Build history of the part. All positions in model axes, mm. A direction names the side the tool comes from. Give positions to 0.01 mm unless a question says otherwise; leave off trailing zeros. Order: outer loops, then holes, each group sorted by start corner. A loop starts at its lowest first (then second) coordinate and runs counter-clockwise, first axis right, second up. Notation, with made-up numbers: (-15, 14) - (37, 14) arc R34 cw to (37, 46) - close; hole circle Ø5 at (38, 50). An arc over 180 degrees is marked (long way). Use a Markdown table: item, result.
from build123d import *

# Parameters (mm, degrees)
F0_W          = 10
F0_H          = 15
F1_DEPTH      = 8
F2_W          = 8
F2_H          = 14
F3_DEPTH      = 14
F5_DEPTH      = 25
F7_DEPTH      = 1
F8_R          = 2
F9_DEPTH      = 1
F10_T1_DEPTH  = 4
F10_S5_W      = 2.04
F10_S5_H      = 2.04
F10_T6_DEPTH  = 2.04
F10_S11_W     = 2.04
F10_S11_H     = 2.04
F10_T12_DEPTH = 2.04
F10_T18_DEPTH = 10
F10_T23_DEPTH = 10
F10_T28_DEPTH = 17
F10_T33_DEPTH = 17
F10_T35_DEPTH = 6
F10_T37_DEPTH = 18
F10_T39_DEPTH = 11
F10_S43_W     = 2.04
F10_S43_H     = 2.04
F10_T44_DEPTH = 2.04
F10_S49_W     = 2.04
F10_S49_H     = 2.04
F10_T50_DEPTH = 2.04


# Not quite as in the source:
# - a fillet or chamfer that OpenCascade refuses, or shapes differently, is made with other operations: its cross-section is extruded or revolved along the edge and cut away or added


with BuildPart() as f1:
    # F0 (on Front) → F1 (new body)
    with BuildSketch(Plane.XZ):
        with Locations((0, 7.5)):
            Rectangle(F0_W, F0_H)
    extrude(amount=F1_DEPTH)

    # F2 (on face) → F3 (cut)
    with BuildSketch(Plane.XZ.offset(8)):
        with Locations((0, 8)):
            Rectangle(F2_W, F2_H)
    extrude(amount=-F3_DEPTH, mode=Mode.SUBTRACT)

    # F4 (on face) → F5 (cut)
    with BuildSketch(Plane(origin=(-5, 0, 0), x_dir=(0, -1, 0), z_dir=(-1, 0, 0))):
        Polygon((8, 15), (1, 15), (8, 1), align=None)
    extrude(amount=-F5_DEPTH, mode=Mode.SUBTRACT)

    # F6 (on face) → F7 (join)
    with BuildSketch(Plane(origin=(0, 0, 0), x_dir=(-1, 0, 0), z_dir=(0, 1, 0))):
        Polygon((4, 15), (5, 15), (2.1132486541, 20), (-2.1132486541, 20), (-5, 15), (-4, 15), (-4, 1), (4, 1), align=None)
    extrude(amount=-F7_DEPTH)

    # F8 (on face) → F9 (join)
    with BuildSketch(Plane.XZ.offset(1)):
        with Locations((0, 17)):
            Circle(F8_R)
    extrude(amount=F9_DEPTH)

    # F10: fillet of radius 2 on 12 edges, made by hand

    # F10_s2 → F10_t1 (join)
    with BuildSketch(Plane.YZ.offset(-2)):
        with BuildLine():
            ThreePointArc((-3, 1), (-1.5857864376, 1.5857864376), (-1, 3))
            Line((-1, 3), (-1, 1))
            Line((-1, 1), (-3, 1))
        make_face()
    extrude(amount=F10_T1_DEPTH)


with BuildPart() as f10_tool4:
    # F10_s5 → F10_t6 (new body)
    with BuildSketch(Plane.XY.offset(3)):
        with Locations((-3.02, -1.98)):
            Rectangle(F10_S5_W, F10_S5_H)
    extrude(amount=-F10_T6_DEPTH)

    # F10_s7 → F10_t8 (revolve, cut)
    with BuildSketch(Plane(origin=(-2, -3, 3), x_dir=(0.7071067812, -0.7071067812, 0), z_dir=(0.7071067812, 0.7071067812, 0))):
        with BuildLine():
            ThreePointArc((0, -2), (2, 0), (0, 2))
            Line((0, 2), (0, -2))
        make_face()
    revolve(axis=Axis((-2, -3, 3), (0, 0, -1)), mode=Mode.SUBTRACT)


with BuildPart() as f1_1:
    add(f1.part)

    # F10_t3: union F10_tool4
    add(f10_tool4.part)


with BuildPart() as f10_tool10:
    # F10_s11 → F10_t12 (new body)
    with BuildSketch(Plane.XY.offset(3)):
        with Locations((3.02, -1.98)):
            Rectangle(F10_S11_W, F10_S11_H)
    extrude(amount=-F10_T12_DEPTH)

    # F10_s13 → F10_t14 (revolve, cut)
    with BuildSketch(Plane(origin=(2, -3, 3), x_dir=(-0.7071067812, -0.7071067812, 0), z_dir=(0.7071067812, -0.7071067812, 0))):
        with BuildLine():
            ThreePointArc((0, -2), (2, 0), (0, 2))
            Line((0, 2), (0, -2))
        make_face()
    revolve(axis=Axis((2, -3, 3), (0, 0, -1)), mode=Mode.SUBTRACT)


with BuildPart() as f1_2:
    add(f1_1.part)

    # F10_t9: union F10_tool10
    add(f10_tool10.part)


with BuildPart() as f10_tool16:
    # F10_s17 → F10_t18 (new body)
    with BuildSketch(Plane.XZ.offset(13)):
        with BuildLine():
            ThreePointArc((-2, 1), (-3.4142135624, 1.5857864376), (-4, 3))
            Line((-4, 3), (-4, 1))
            Line((-4, 1), (-2, 1))
        make_face()
    extrude(amount=-F10_T18_DEPTH)

    split(bisect_by=Plane(origin=(0, -6.8, 3.4), x_dir=(1, 0, 0), z_dir=(0, 0.894427191, -0.4472135955)), keep=Keep.TOP)


with BuildPart() as f1_3:
    add(f1_2.part)

    # F10_t15: union F10_tool16
    add(f10_tool16.part)


with BuildPart() as f10_tool21:
    # F10_s22 → F10_t23 (new body)
    with BuildSketch(Plane.XZ.offset(13)):
        with BuildLine():
            ThreePointArc((2, 1), (3.4142135624, 1.5857864376), (4, 3))
            Line((4, 3), (4, 1))
            Line((4, 1), (2, 1))
        make_face()
    extrude(amount=-F10_T23_DEPTH)

    split(bisect_by=Plane(origin=(0, -6.8, 3.4), x_dir=(1, 0, 0), z_dir=(0, 0.894427191, -0.4472135955)), keep=Keep.TOP)


with BuildPart() as f1_4:
    add(f1_3.part)

    # F10_t20: union F10_tool21
    add(f10_tool21.part)


with BuildPart() as f10_tool26:
    # F10_s27 → F10_t28 (new body)
    with BuildSketch(Plane.XY.offset(20)):
        with BuildLine():
            ThreePointArc((2, -1), (3.4142135624, -1.5857864376), (4, -3))
            Line((4, -3), (4, -1))
            Line((4, -1), (2, -1))
        make_face()
    extrude(amount=-F10_T28_DEPTH)

    split(bisect_by=Plane(origin=(0, -6.8, 3.4), x_dir=(1, 0, 0), z_dir=(0, 0.894427191, -0.4472135955)), keep=Keep.TOP)


with BuildPart() as f1_5:
    add(f1_4.part)

    # F10_t25: union F10_tool26
    add(f10_tool26.part)


with BuildPart() as f10_tool31:
    # F10_s32 → F10_t33 (new body)
    with BuildSketch(Plane.XY.offset(3)):
        with BuildLine():
            ThreePointArc((-4, -3), (-3.4142135624, -1.5857864376), (-2, -1))
            Line((-2, -1), (-4, -1))
            Line((-4, -1), (-4, -3))
        make_face()
    extrude(amount=F10_T33_DEPTH)

    split(bisect_by=Plane(origin=(0, -6.8, 3.4), x_dir=(1, 0, 0), z_dir=(0, 0.894427191, -0.4472135955)), keep=Keep.TOP)


with BuildPart() as f1_6:
    add(f1_5.part)

    # F10_t30: union F10_tool31
    add(f10_tool31.part)

    # F10_s36 → F10_t35 (cut)
    with BuildSketch(Plane.YZ.offset(-3)):
        with BuildLine():
            ThreePointArc((-2, 0), (-0.5857864376, 0.5857864376), (0, 2))
            Line((0, 2), (0, 0))
            Line((0, 0), (-2, 0))
        make_face()
    extrude(amount=F10_T35_DEPTH, mode=Mode.SUBTRACT)

    # F10_s38 → F10_t37 (cut)
    with BuildSketch(Plane.XY.offset(2)):
        with BuildLine():
            ThreePointArc((-5, -2), (-4.4142135624, -0.5857864376), (-3, 0))
            Line((-3, 0), (-5, 0))
            Line((-5, 0), (-5, -2))
        make_face()
        with BuildLine():
            ThreePointArc((5, -2), (4.4142135624, -0.5857864376), (3, 0))
            Line((3, 0), (5, 0))
            Line((5, 0), (5, -2))
        make_face()
    extrude(amount=F10_T37_DEPTH, mode=Mode.SUBTRACT)

    # F10_s40 → F10_t39 (cut)
    with BuildSketch(Plane.XZ.offset(2)):
        with BuildLine():
            ThreePointArc((-5, 2), (-4.4142135624, 0.5857864376), (-3, 0))
            Line((-3, 0), (-5, 0))
            Line((-5, 0), (-5, 2))
        make_face()
        with BuildLine():
            ThreePointArc((5, 2), (4.4142135624, 0.5857864376), (3, 0))
            Line((3, 0), (5, 0))
            Line((5, 0), (5, 2))
        make_face()
    extrude(amount=F10_T39_DEPTH, mode=Mode.SUBTRACT)


with BuildPart() as f10_tool42:
    # F10_s43 → F10_t44 (new body)
    with BuildSketch(Plane.YZ.offset(-3)):
        with Locations((-0.98, 0.98)):
            Rectangle(F10_S43_W, F10_S43_H)
    extrude(amount=-F10_T44_DEPTH)

    # F10_s45 → F10_t46 (revolve, cut)
    with BuildSketch(Plane(origin=(-3, -2, 2), x_dir=(0, -0.7071067812, 0.7071067812), z_dir=(0, -0.7071067812, -0.7071067812))):
        with BuildLine():
            ThreePointArc((0, -2), (2, 0), (0, 2))
            Line((0, 2), (0, -2))
        make_face()
    revolve(axis=Axis((-3, -2, 2), (-1, 0, 0)), mode=Mode.SUBTRACT)


with BuildPart() as f1_7:
    add(f1_6.part)

    # F10_t41: cut F10_tool42
    add(f10_tool42.part, mode=Mode.SUBTRACT)


with BuildPart() as f10_tool48:
    # F10_s49 → F10_t50 (new body)
    with BuildSketch(Plane.YZ.offset(3)):
        with Locations((-0.98, 0.98)):
            Rectangle(F10_S49_W, F10_S49_H)
    extrude(amount=F10_T50_DEPTH)

    # F10_s51 → F10_t52 (revolve, cut)
    with BuildSketch(Plane(origin=(3, -2, 2), x_dir=(0, -0.7071067812, 0.7071067812), z_dir=(0, 0.7071067812, 0.7071067812))):
        with BuildLine():
            ThreePointArc((0, -2), (2, 0), (0, 2))
            Line((0, 2), (0, -2))
        make_face()
    revolve(axis=Axis((3, -2, 2), (1, 0, 0)), mode=Mode.SUBTRACT)


with BuildPart() as f1_8:
    add(f1_7.part)

    # F10_t47: cut F10_tool48
    add(f10_tool48.part, mode=Mode.SUBTRACT)


solid = f1_8.part
1) Slice it at C-C (x = 0). Write the cut outline in (y, z).
Computed:
| item | result |
|---|---|
| outline | (-8, 0) - (-2, 0) arc R2 ccw to (0, 2) - (0, 20) - (-1, 20) - (-1, 19) - (-2, 19) - (-2, 15) - (-1, 15) - (-1, 3) arc R2 cw to (-3, 1) - (-8, 1) - close |
2) Slice it at D-D (z = 13.75). Write the cut outline in (x, y) (3 decimals).
Computed:
| item | result |
|---|---|
| outline | (-4.965, -1.625) - (-3.452, -1.625) arc R2 cw to (-2, -1) - (2, -1) arc R2 cw to (3.452, -1.625) - (4.965, -1.625) arc R2 ccw to (3, 0) - (-3, 0) arc R2 ccw to start |
3) Two-plate mould, pull along X, no slides. Class faces 1 (the flat face through (-5, -4, 6)), 2 (the flat face through (0, -1, 14)), 3 (the cylindrical face through (4.43, -0.6, 8.29)): +X half, -X half, draft (parallel to the pull), parting line (faces both ways), or undercut.
Computed:
| item | result |
|---|---|
| face 1 | -X half |
| face 2 | undercut |
| face 3 | +X half |
4) Pin check, flat tips, straight feed: P1, Ø1, axis at y = -6, z = 6.5, coming from the +X side; P2, Ø3, axis at x = 0, y = -4.5, coming from the +Z side; P3, Ø1, axis at x = -4, z = 5.5, coming from the +Y side; P4, Ø6, axis at x = 3.5, z = 4.5, coming from the -Y side. Stop position of each tip, or through.
Computed:
| item | result |
|---|---|
| P1 | passes through |
| P2 | stops at z = 1 |
| P3 | stops at y = -0.06 |
| P4 | stops at y = -7.75 |
5) Tool access for faces 4 (the flat face through (0, -2, 17)), 5 (the cylindrical face through (-0.26, -1.493, 18.983)), 6 (the flat face through (4, -4, 5)): list every direction of +Z, -Z, +X, -X, +Y, -Y with a clear straight run to the whole face (end or side of a thin tool).
Computed:
| item | result |
|---|---|
| face 4 | +Z, +X, -X, -Y |
| face 5 | -Y |
| face 6 | +Z, -Y |
6) Slice it at B-B (z = 17). Write the cut outline in (x, y).
Computed:
| item | result |
|---|---|
| outline | (-3.85, -1) - (-2, -1) - (-2, -2) - (2, -2) - (2, -1) - (3.85, -1) - (3.85, -0.19) arc R2 ccw to (3, 0) - (-3, 0) arc R2 ccw to (-3.85, -0.19) - close |
7) Slice it at A-A (y = -4.5). Write the cut outline in (x, z), and give its area (3 significant figures).
Computed:
| item | result |
|---|---|
| outline | (-5, 2) arc R2 ccw to (-3, 0) - (3, 0) arc R2 ccw to (5, 2) - (5, 8) - (4, 8) - (4, 3) arc R2 cw to (2, 1) - (-2, 1) arc R2 cw to (-4, 3) - (-4, 8) - (-5, 8) - close |
| area | 24.0 mm² |
8) Wall check: line 1 (Y direction, x = 1.75, z = 16.5); line 2 (Z direction, x = 1.5, y = -5); line 3 (Y direction, x = -0.5, z = 5.5). Give the ranges that are in metal, low to high. Write a range as from..to.
Computed:
| item | result |
|---|---|
| line 1 | y = -2..0 |
| line 2 | z = 0..1 |
| line 3 | y = -1..0 |
